Check sheet for the drawn part. Datum: minimum x, y, z corner. Units: mm. Give positions to 0.01 mm unless a question says otherwise; leave off trailing zeros. Order: outer loops, then holes, each group sorted by start corner. A loop starts at its lowest first (then second) coordinate and runs counter-clockwise, first axis right, second up.
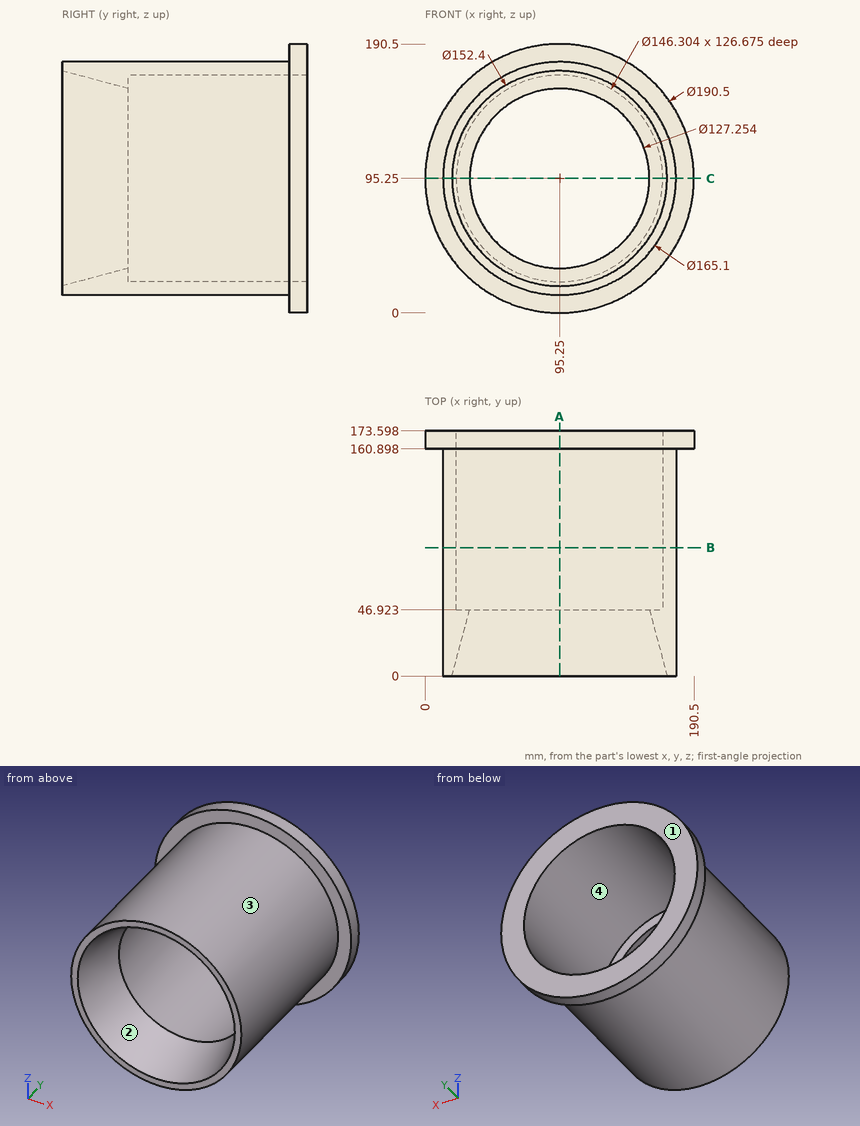
(1) Go/stop test with flat-tipped pins: pin 1 (3 mm diameter, centred on x = 81.5, y = 82.5, fed in from +Z); pin 2 (4 mm diameter, centred on y = 142, z = 34.5, fed in from -X); pin 3 (8 mm diameter, centred on y = 143, z = 52, fed in from +X). Record where each tip stops, or that it passes through.
Solved:
pin 1: stops at z = 176.89
pin 2: stops at x = 37.26
pin 3: stops at x = 167.87
(2) Release check for a two-part mould opening along Z. For the marked faces 1, 2, 3 and 4 record: pulls with the +Z half, pulls with the -Z half, needs draft (parallel to the pull), parting line crosses it, or undercut.
Solved:
face 1: needs draft
face 2: undercut
face 3: parting line crosses it
face 4: undercut
(3) Scan lines: line 1 (X direction, y = 117.5, z = 95.25); line 2 (Y direction, x = 56, z = 10.5). Record each from-to range of solid material in increasing order.
Solved:
line 1: x = 12.7 to 22.1, 168.4 to 177.8
line 2: y = 160.9 to 173.6
(4) Section check B-B, the plane y = 91. Enter the section's corners in (x, z), then the cut area to 3 significant figures.
Solved:
outline: circle Ø165.1 at (95.25, 95.25); hole circle Ø146.3 at (95.25, 95.25)
area: 4,600 mm2
(5) Section check C-C, the plane z = 95.25. Enter the section's corners in (x, y).
Solved:
outline: (0, 160.9) - (12.7, 160.9) - (12.7, 0) - (19.05, 0) - (31.62, 46.92) - (22.1, 46.92) - (22.1, 173.6) - (0, 173.6) - close; (158.88, 46.92) - (171.45, 0) - (177.8, 0) - (177.8, 160.9) - (190.5, 160.9) - (190.5, 173.6) - (168.4, 173.6) - (168.4, 46.92) - close
(6) Section check A-A, the plane x = 95.25. Enter the section's corners in (y, z).
Solved:
outline: (0, 12.7) - (160.9, 12.7) - (160.9, 0) - (173.6, 0) - (173.6, 22.1) - (46.92, 22.1) - (46.92, 31.62) - (0, 19.05) - close; (0, 171.45) - (46.92, 158.88) - (46.92, 168.4) - (173.6, 168.4) - (173.6, 190.5) - (160.9, 190.5) - (160.9, 177.8) - (0, 177.8) - close
